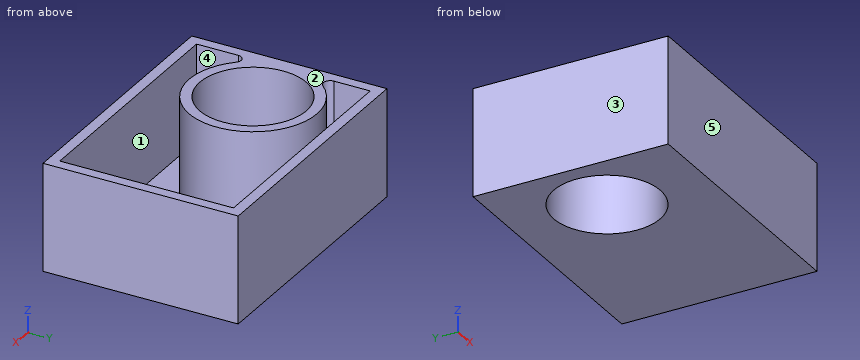
```python
from build123d import *

# Parameters (mm, degrees)
F0_W     = 62.6746565104
F0_H     = 46.1766123772
F0_R     = 12.6048441678
F1_DEPTH = 25.4
F2_T     = -2.54
F3_R     = 1.5875


with BuildPart() as f1:
    # F0 (on Top) → F1 (new body)
    with BuildSketch(Plane.XY):
        with Locations((31.3373282552, 23.0883061886)):
            Rectangle(F0_W, F0_H)
        with Locations((16.4661593735, 23.7301085144)):
            Circle(F0_R, mode=Mode.SUBTRACT)
    extrude(amount=F1_DEPTH)

    # F2
    f2_openings = [f1.faces().sort_by_distance(p)[0] for p in [
        (34.436685, 22.954546, 25.4),
    ]]
    offset(amount=F2_T, openings=f2_openings)

    # F3
    f3_edges = [f1.edges().sort_by_distance(p)[0] for p in [
        (2.54, 29.682284, 13.97),
        (2.54, 17.777933, 13.97),
    ]]
    fillet(f3_edges, radius=F3_R)


solid = f1.part
```
Check sheet for the modelled part. Datum: model origin and axes. Units: mm. Face numbers are marked on the shaded views. A direction names the side the tool comes from. Coordinates: 2 decimals unless noted, no trailing zeros. Write each loop counter-clockwise with the first axis right and the second up, starting at its lowest first coordinate (ties: lowest second). Pieces come first, ordered by that corner, then holes. Notation, with made-up numbers: M 34.5,41 L 92.5,41 A20 ccw 92.5,70 Z; hole C 85,-34.5 d1. An arc over 180 degrees is marked long. Write item = value, one per line. Start each with the question number.
1. Sectioned sample at B-B (y = 7). Record the cut outline in (x, z).
2. Thickness scan on probe 1 along Y at (x, z) = (16.5, 10.25); probe 2 along X at (y, z) = (23.5, 23); probe 3 along X at (y, z) = (42, 12.25). Record the ranges inside material, lowest first.
3. Sectioned sample at A-A (x = 8.5). Record the cut outline in (y, z), then the cut area to 3 significant figures.
4. Mould release check, pull along X, two halves, no side actions. Record for the marked faces 3, 4 and 5: pulls with the +X half, pulls with the -X half, needs draft (parallel to the pull), parting line crosses it, or undercut.
5. Go/stop test with flat-tipped pins: pin 1 (1 mm diameter, centred on x = 30, z = 13.5, fed in from -Y); pin 2 (4 mm diameter, centred on x = 9.5, y = 5.5, fed in from +Z). Record where each tip stops, or that it passes through.
6. Sectioned sample at D-D (y = 22.5). Record the cut outline in (x, z).
7. Sectioned sample at C-C (x = 34). Record the cut outline in (y, z).
8. Tool access check on the marked faces 1 and 2. Record the directions out of +Z, -Z, +X, -X, +Y, -Y that give a thin tool (end or side, any length) a straight path to the whole face; none if there is none.
The answers:
q1.outline = M 0,0 L 62.67,0 L 62.67,25.4 L 60.13,25.4 L 60.13,2.54 L 2.54,2.54 L 2.54,25.4 L 0,25.4 Z
q2.probe_1 = 0 to 2.54, 8.59 to 11.13, 36.33 to 38.87, 43.64 to 46.18
q2.probe_2 = 0 to 3.86, 29.07 to 31.61, 60.13 to 62.67
q2.probe_3 = 0 to 2.54, 60.13 to 62.67
q3.outline = M 0,0 L 13.96,0 L 13.96,25.4 L 10.85,25.4 L 10.85,2.54 L 2.54,2.54 L 2.54,25.4 L 0,25.4 Z; M 33.5,0 L 46.18,0 L 46.18,25.4 L 43.64,25.4 L 43.64,2.54 L 36.61,2.54 L 36.61,25.4 L 33.5,25.4 Z
q3.area = 326 mm²
q4.face_3 = pulls with the -X half
q4.face_4 = undercut
q4.face_5 = needs draft
q5.pin_1 = 0
q5.pin_2 = 2.54
q6.outline = M 0,0 L 3.92,0 L 3.92,25.4 L 0,25.4 Z; M 29.01,0 L 62.67,0 L 62.67,25.4 L 60.13,25.4 L 60.13,2.54 L 31.56,2.54 L 31.56,25.4 L 29.01,25.4 Z
q7.outline = M 0,0 L 46.18,0 L 46.18,25.4 L 43.64,25.4 L 43.64,2.54 L 2.54,2.54 L 2.54,25.4 L 0,25.4 Z
q8.face_1 = +Z
q8.face_2 = +Z, +X, -X, +Y, -Y
